CAD build for the part. Positions are in the model's coordinates, mm. A direction names the side the tool comes from. Give positions to 0.01 mm unless a question says otherwise; leave off trailing zeros. Write each loop counter-clockwise with the first axis right and the second up, starting at its lowest first coordinate (ties: lowest second). Pieces come first, ordered by that corner, then holes. Notation, with made-up numbers: (-15, 33) -> (27, 33) arc R19 ccw to (27, 41) -> close; hole circle Ø11 at (61.5, 67). An arc over 180 degrees is marked (long way). Answer as a JSON object with one key per item and string values.
```python
from build123d import *

# Parameters (mm, degrees)
SKETCH_W        = 49
SKETCH_H        = 49
PAD_DEPTH       = 18
POCKET_DEPTH    = 47
SKETCH002_W     = 14
SKETCH002_H     = 25
POCKET001_DEPTH = 5
SKETCH003_W     = 16
SKETCH003_H     = 46.5
POCKET002_DEPTH = 3
SKETCH004_W     = 2.9
SKETCH004_H     = 15
PAD001_DEPTH    = 16
SKETCH005_R     = 2.5
POCKET003_DEPTH = 20.801
POCKET004_DEPTH = 5
POCKET005_DEPTH = 5
FILLET_R        = 7.4
SKETCH008_R     = 4
POCKET006_DEPTH = 5


with BuildPart() as part:
    # Sketch → Pad (new body)
    with BuildSketch(Plane.XZ):
        with Locations((24.5, 24.5)):
            Rectangle(SKETCH_W, SKETCH_H)
    extrude(amount=PAD_DEPTH)

    # Sketch001 (on Face1 of Pad) → Pocket (cut)
    with BuildSketch(Plane(origin=(0, 0, 49), x_dir=(-1, 0, 0), z_dir=(0, 0, 1))):
        with BuildLine():
            Line((-47, 16), (-2, 16))
            ThreePointArc((-2, 2), (-1, 9), (-2, 16))
            Line((-2, 2), (-47, 2))
            ThreePointArc((-47, 16), (-48, 9), (-47, 2))
        make_face()
    extrude(amount=-POCKET_DEPTH, mode=Mode.SUBTRACT)

    # Sketch002 (on Face4 of Pocket) → Pocket001 (cut)
    with BuildSketch(Plane.XZ.offset(18)):
        with Locations((14.5, 24.5)):
            Rectangle(SKETCH002_W, SKETCH002_H)
    extrude(amount=-POCKET001_DEPTH, mode=Mode.SUBTRACT)

    # Sketch003 (on Face3 of Pocket001) → Pocket002 (cut)
    with BuildSketch(Plane(origin=(0, 0, 0), x_dir=(1, 0, 0), z_dir=(0, 1, 0))):
        with Locations((8, -25.75)):
            Rectangle(SKETCH003_W, SKETCH003_H)
    extrude(amount=-POCKET002_DEPTH, mode=Mode.SUBTRACT)

    # Sketch004 (on Face10 of Pocket002) → Pad001 (join)
    with BuildSketch(Plane.XZ.offset(18)):
        with Locations((29.65, 7.5)):
            Rectangle(SKETCH004_W, SKETCH004_H)
        with Locations((35.55, 7.5)):
            Rectangle(SKETCH004_W, SKETCH004_H)
    extrude(amount=PAD001_DEPTH)

    # Sketch005 (on Face19 of Pad001) → Pocket003 (cut, through all)
    with BuildSketch(Plane(origin=(28.2, 0, 0), x_dir=(0, 0, -1), z_dir=(-1, 0, 0))):
        with Locations((-7.5, 26.5)):
            Circle(SKETCH005_R)
    extrude(amount=-POCKET003_DEPTH, mode=Mode.SUBTRACT)

    # Sketch006 (on Face9 of Pocket003) → Pocket004 (cut)
    with BuildSketch(Plane(origin=(49, 0, 0), x_dir=(0, 0, 1), z_dir=(1, 0, 0))):
        with BuildLine():
            ThreePointArc((19.5, 13.5), (15, 9), (19.5, 4.5))
            Line((19.5, 4.5), (29.5, 4.5))
            ThreePointArc((29.5, 4.5), (34, 9), (29.5, 13.5))
            Line((29.5, 13.5), (19.5, 13.5))
        make_face()
    extrude(amount=-POCKET004_DEPTH, mode=Mode.SUBTRACT)

    # Sketch007 (on Face11 of Pocket004) → Pocket005 (cut)
    with BuildSketch(Plane(origin=(0, 0, 0), x_dir=(0, 0, -1), z_dir=(-1, 0, 0))):
        with BuildLine():
            ThreePointArc((-40, 13.5), (-44.5, 9), (-40, 4.5))
            Line((-40, 4.5), (-34, 4.5))
            ThreePointArc((-34, 4.5), (-29.5, 9), (-34, 13.5))
            Line((-34, 13.5), (-40, 13.5))
        make_face()
    extrude(amount=-POCKET005_DEPTH, mode=Mode.SUBTRACT)

    # Fillet
    fillet_edges = [part.edges().sort_by_distance(p)[0] for p in [
        (29.65, -34, 15),
        (35.55, -34, 15),
        (35.55, -34, 0),
        (29.65, -34, 0),
    ]]
    fillet(fillet_edges, radius=FILLET_R)

    # Sketch008 (on Face11 of Fillet) → Pocket006 (cut)
    with BuildSketch(Plane(origin=(0, 0, 0), x_dir=(0, 0, -1), z_dir=(-1, 0, 0))):
        with Locations((-24.5, 9)):
            Circle(SKETCH008_R)
    extrude(amount=-POCKET006_DEPTH, mode=Mode.SUBTRACT)


solid = part.part
```
1) Pin check, flat tips, straight feed: pin 1 (11 mm diameter, centred on x = 27, y = -8, fed in from +Z); pin 2 (10 mm diameter, centred on x = 7, z = 31, fed in from -Y); pin 3 (0.9 mm diameter, centred on x = 29, y = -23, fed in from +Z); pin 4 (3 mm diameter, centred on y = -26.5, z = 7.5, fed in from +X). Stop position of each tip, or through.
Model answer:
{"pin 1": "stops at z = 2", "pin 2": "stops at y = -18", "pin 3": "stops at z = 15", "pin 4": "passes through"}
2) Slice it at B-B (z = 24). List the corners of the cut face in (x, y).
Model answer:
{"outline": "(0, -18) -> (7.5, -18) -> (7.5, -16) -> (2, -16) arc R25 cw to (1.32, -12.97) -> (0, -12.97) -> close; (0, -5.03) -> (1.32, -5.03) arc R25 cw to (1.73, -3) -> (0, -3) -> close; (16, -2) -> (47, -2) arc R25 cw to (47.59, -4.5) -> (49, -4.5) -> (49, 0) -> (16, 0) -> close; (21.5, -18) -> (49, -18) -> (49, -13.5) -> (47.59, -13.5) arc R25 cw to (47, -16) -> (21.5, -16) -> close"}
3) Wall check: probe 1 along Y at (x, z) = (36.35, 7.5); probe 2 along Z at (x, y) = (0.85, -9); probe 3 along X at (y, z) = (-27, 14). Give the ranges that are in metal, low to high.
Model answer:
{"probe 1": "y = -34 to -29, -24 to -16, -2 to 0", "probe 2": "z = 0 to 20.5, 28.5 to 29.5, 44.5 to 49", "probe 3": "x = 28.2 to 31.1, 34.1 to 37"}
4) Slice it at A-A (y = -9). List the corners of the cut face in (x, z).
Model answer:
{"outline": "(0, 0) -> (49, 0) -> (49, 15) -> (48, 15) -> (48, 2) -> (1, 2) -> (1, 20.5) -> (0, 20.5) -> close; (0, 28.5) -> (1, 28.5) -> (1, 29.5) -> (0, 29.5) -> close; (0, 44.5) -> (1, 44.5) -> (1, 49) -> (0, 49) -> close; (48, 34) -> (49, 34) -> (49, 49) -> (48, 49) -> close"}
5) 3-axis set-ups, long thin cutter, end or side, ignore diameter. For faces 1 (the flat face through (36, -22, 15)), 2 (the cylindrical face through (48.5, -8.9, 34)), 3 (the cylindrical face through (0.5, -8.9, 29.5)), 4 (the flat face through (14, -17, 12)), 5 (the flat face through (7.5, -17, 24)): which of +Z, -Z, +X, -X, +Y, -Y reach the whole face in a straight line?
Model answer:
{"face 1": "+Z, +X, -X, -Y", "face 2": "+X", "face 3": "-X", "face 4": "-Y", "face 5": "+Y, -Y"}
6) Slice it at C-C (x = 38.5). List the corners of the cut face in (y, z).
Model answer:
{"outline": "(-18, 0) -> (0, 0) -> (0, 49) -> (-2, 49) -> (-2, 2) -> (-16, 2) -> (-16, 49) -> (-18, 49) -> close"}
7) Slice it at D-D (z = 43). List the corners of the cut face in (x, y).
Model answer:
{"outline": "(0, -18) -> (49, -18) -> (49, 0) -> (16, 0) -> (16, -2) -> (47, -2) arc R25 cw to (47, -16) -> (2, -16) arc R25 cw to (1.23, -12.35) -> (0, -12.35) -> close; (0, -5.65) -> (1.23, -5.65) arc R25 cw to (1.73, -3) -> (0, -3) -> close"}
8) Mould opens along Y. For faces 6 (the cylindrical face through (0.5, -9.1, 44.5)), 7 (the flat face through (14, -17, 37)), 8 (the cylindrical face through (35.57, -31.775, 2.11)), 9 (the flat face through (24, -9, 2)) say: released by +Y, released by -Y, zero draft, split by the parting line, or undercut.
Model answer:
{"face 6": "undercut", "face 7": "zero draft", "face 8": "released by -Y", "face 9": "undercut"}
